Read the model definition and answer for the solid it produces. Units are mm, in the model's axes. A direction names the side the tool comes from. Give positions to 0.01 mm unless a question says otherwise; leave off trailing zeros. Loops run counter-clockwise (first coordinate to the right, second up) from the corner with the lowest first, then second, coordinate; pieces in that order, holes last. Notation, with made-up numbers: (64, 4.5) - (110, 4.5) arc R16 cw to (110, 9.5) - close; hole circle Ø2 at (62, 20.5). An arc over 180 degrees is marked (long way). Write each question's results on one line, items separated by ' | '. Start each with the question number.
Q1. The part is cut by section A-A, the plane z = 11. Write down the section's boundary in (x, y) (3 decimals), plus the area to 3 significant figures.
Q2. The part is cut by section B-B, the plane x = -11.5. Write down the section's boundary in (y, z) (3 decimals), plus the area to 3 significant figures.
Q3. The part is cut by section C-C, the plane y = 24. Write down the section's boundary in (x, z).
Q4. Given pin 1 (3 mm diameter, centred on y = -4.5, z = 4.5, fed in from -X); pin 2 (6 mm diameter, centred on y = 31.5, z = 18, fed in from -X); pin 3 (1.5 mm diameter, centred on x = 0, z = 21.5, fed in from +Y), each flat-ended and moving along its own axis, determine where each tip first touches the part or whether it passes through.
Q5. Find the intervals of material crossed by line 1 (Y direction, x = -9.5, z = 3.75) (3 decimals); line 2 (X direction, y = -24, z = 6.25); line 3 (Y direction, x = 34, z = 3.25), in increasing order. Write a range as from..to.
Q6. For faces 1 (the flat face through (-36, 57.15, 13)), 2 (the flat face through (-63.5, 59, 13)), determine the directions among +Z, -Z, +X, -X, +Y, -Y from which every point of the face is accessible in a straight line to the end or side of a thin tool.
```python
from build123d import *

# Parameters (mm, degrees)
BOSS_EXTRUDE1_DEPTH = 25.4
CUT_EXTRUDE1_DEPTH  = 165.4


with BuildPart() as part:
    # Sketch1 → Boss-Extrude1 (new body)
    with BuildSketch(Plane.XY):
        with BuildLine():
            ThreePointArc((5.857864376, 51.292135624), (-0.6306026, 55.62759065), (-8.284271247, 57.15))
            Line((-8.284271247, 57.15), (-63.5, 57.15))
            Line((-63.5, 57.15), (-63.5, 60.325))
            Line((-63.5, 60.325), (-6.969143187, 60.325))
            ThreePointArc((-6.969143187, 60.325), (0.68452546, 58.80259065), (7.172992437, 54.467135624))
            Line((7.172992437, 54.467135624), (6.735192091, 54.90493597))
            Line((6.735192091, 54.90493597), (54.90493597, 6.735192091))
            Line((54.90493597, 6.735192091), (55.397071593, 6.243056467))
            ThreePointArc((55.397071593, 6.243056467), (59.73252662, -0.245410509), (61.25493597, -7.899079157))
            Line((61.25493597, -7.899079157), (61.25493597, -58.192189171))
            Line((61.25493597, -58.192189171), (60.059609459, -58.192189171))
            Line((60.059609459, -58.192189171), (57.534761691, -7.695233822))
            ThreePointArc((57.534761691, -7.695233822), (55.840378599, -0.581197787), (51.701850537, 5.448149463))
            Line((51.701850537, 5.448149463), (5.857864376, 51.292135624))
        make_face()
    extrude(amount=BOSS_EXTRUDE1_DEPTH)

    # Sketch2 → Cut-Extrude1 (cut)
    with BuildSketch(Plane(origin=(61.25493597, 0, 0), x_dir=(0, 0, -1), z_dir=(1, 0, 0))):
        Polygon((-25.4, 54.467135624), (-20.4, -58.192189171), (-53.926173028, -59.680134048), align=None)
        Polygon((0, 54.467135624), (-5, -58.192189171), (16.325141492, -58.192189171), align=None)
    extrude(amount=-CUT_EXTRUDE1_DEPTH, mode=Mode.SUBTRACT)


solid = part.part
```
Check sheet entries:
1) outline: (-63.5, 57.15) - (-8.284, 57.15) arc R20 cw to (5.858, 51.292) - (51.702, 5.448) arc R20 cw to (57.535, -7.695) - (60.06, -58.192) - (61.255, -58.192) - (61.255, -7.899) arc R20 ccw to (55.397, 6.243) - (7.173, 54.467) arc R20 ccw to (-6.969, 60.325) - (-63.5, 60.325) - close | area: 620 mm^2
2) outline: (57.15, 0) - (60.325, 0) - (60.325, 25.4) - (57.15, 25.4) - close | area: 80.6 mm^2
3) outline: (33.15, 1.35) - (37.64, 1.35) - (37.64, 24.05) - (33.15, 24.05) - close
4) pin 1: stops at x = 56.73 | pin 2: stops at x = 22.65 | pin 3: stops at y = 59.33
5) line 1: y = 57.15..60.325 | line 2: x = 58.35..61.25 | line 3: y = 23.15..27.64
6) face 1: +Z, -Z, -X, -Y | face 2: +Z, -Z, -X, +Y, -Y
